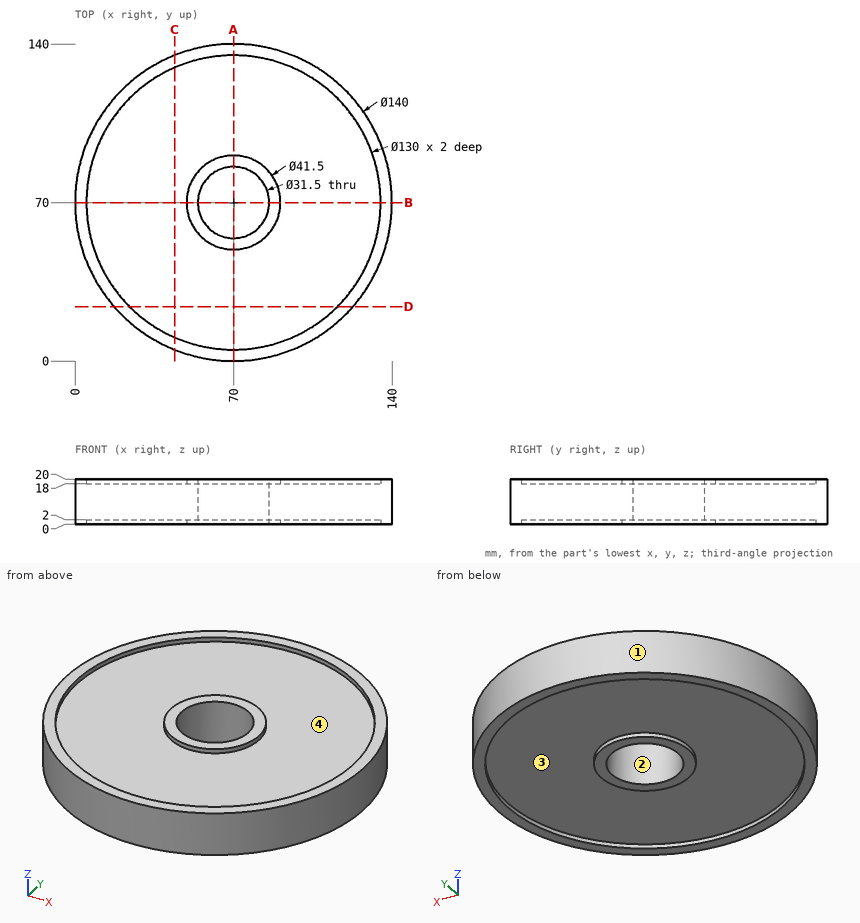
Print and shaded views of the part. All mm, measured from the part's lowest x, y and z. A direction names the side the tool comes from. Coordinates: 2 decimals unless noted, no trailing zeros. Order: outer loops, then holes, each group sorted by start corner. A loop starts at its lowest first (then second) coordinate and runs counter-clockwise, first axis right, second up.
(1) Slice it at C-C, the plane x = 44. Write the cut outline in (y, z).
Check sheet entries:
outline: (5.01, 0) - (10.43, 0) - (10.43, 2) - (129.57, 2) - (129.57, 0) - (134.99, 0) - (134.99, 20) - (129.57, 20) - (129.57, 18) - (10.43, 18) - (10.43, 20) - (5.01, 20) - close
(2) Pull direction X, two halves, no side cores. Call the marked faces 1 and 2: pulls with the +X half, pulls with the -X half, needs draft (parallel to the pull), parting line crosses it, or undercut.
Check sheet entries:
face 1: parting line crosses it
face 2: undercut
(3) Slice it at D-D, the plane y = 24. Write the cut outline in (x, z), and give its area (3 significant figures).
Check sheet entries:
outline: (17.24, 0) - (24.08, 0) - (24.08, 2) - (115.92, 2) - (115.92, 0) - (122.76, 0) - (122.76, 20) - (115.92, 20) - (115.92, 18) - (24.08, 18) - (24.08, 20) - (17.24, 20) - close
area: 1,740 mm2
(4) Pin check, flat tips, straight feed: pin 1 Ø1.5 at (y, z) = (105, 6) entering from +X; pin 2 Ø6 at (y, z) = (82, 15.5) entering from -X; pin 3 Ø4 at (y, z) = (84, 10.5) entering from +X. Stop position of each tip, or through.
Check sheet entries:
pin 1: stops at x = 131.05
pin 2: stops at x = 0.58
pin 3: stops at x = 138.96
(5) Tool access for the marked faces 3 and 4: list every direction of +Z, -Z, +X, -X, +Y, -Y with a clear straight run to the whole face (end or side of a thin tool).
Check sheet entries:
face 3: -Z
face 4: +Z
(6) Probe L1, parallel to Y at x = 70, z = 0.5; L2, parallel to Y at x = 70, z = 4.5; L3, parallel to Y at x = 29.5, z = 1.5. List the from-to ranges inside material, lowest first.
Check sheet entries:
L1: y = 0 to 5, 49.25 to 54.25, 85.75 to 90.75, 135 to 140
L2: y = 0 to 54.25, 85.75 to 140
L3: y = 12.91 to 19.16, 120.84 to 127.09
(7) Slice it at A-A, the plane x = 70. Write the cut outline in (y, z).
Check sheet entries:
outline: (0, 0) - (5, 0) - (5, 2) - (49.25, 2) - (49.25, 0) - (54.25, 0) - (54.25, 20) - (49.25, 20) - (49.25, 18) - (5, 18) - (5, 20) - (0, 20) - close; (85.75, 0) - (90.75, 0) - (90.75, 2) - (135, 2) - (135, 0) - (140, 0) - (140, 20) - (135, 20) - (135, 18) - (90.75, 18) - (90.75, 20) - (85.75, 20) - close
